from build123d import *

# Parameters (mm, degrees)
F0_W     = 43.18
F0_H     = 21.971
F0_W_2   = 40.64
F0_H_2   = 19.431
F1_DEPTH = 16.1544
F0_W_3   = 37.592
F0_H_3   = 16.383
F2_DEPTH = 1.27
F3_R     = 1.27
F4_R     = 1.27
F5_R     = 1.785938
F6_DEPTH = 7.62
F7_R     = 1.785938
F8_DEPTH = 7.62


with BuildPart() as f1:
    # F0 (on Front) → F1 (new body)
    with BuildSketch(Plane.XZ):
        Rectangle(F0_W, F0_H)
        Rectangle(F0_W_2, F0_H_2, mode=Mode.SUBTRACT)
    extrude(amount=F1_DEPTH)

    # F0 (on Front) → F2 (join)
    with BuildSketch(Plane.XZ):
        Rectangle(F0_W_2, F0_H_2)
        Rectangle(F0_W_3, F0_H_3, mode=Mode.SUBTRACT)
    extrude(amount=F2_DEPTH)

    # F3
    f3_edges = [f1.edges().sort_by_distance(p)[0] for p in [
        (-21.59, -8.0772, 10.9855),
        (-21.59, -8.0772, -10.9855),
        (21.59, -8.0772, -10.9855),
        (21.59, -8.0772, 10.9855),
    ]]
    fillet(f3_edges, radius=F3_R)

    # F4
    f4_edges = [f1.edges().sort_by_distance(p)[0] for p in [
        (0, 0, -10.9855),
    ]]
    fillet(f4_edges, radius=F4_R)

    # F5 (on face) → F6 (cut)
    with BuildSketch(Plane.YZ.offset(21.59)):
        with Locations((-8.7122, 0)):
            Circle(F5_R)
    extrude(amount=-F6_DEPTH, mode=Mode.SUBTRACT)

    # F7 (on face) → F8 (cut)
    with BuildSketch(Plane(origin=(-21.59, 0, 0), x_dir=(0, -1, 0), z_dir=(-1, 0, 0))):
        with Locations((8.7122, 0)):
            Circle(F7_R)
    extrude(amount=-F8_DEPTH, mode=Mode.SUBTRACT)


solid = f1.part
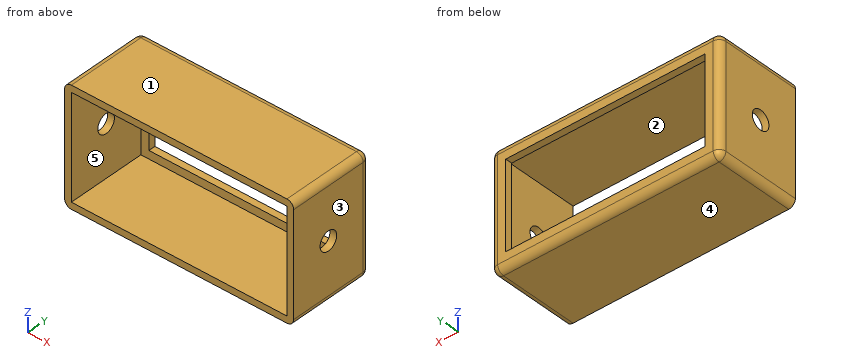
Work out the finished part from the listing and answer in its coordinate system (mm). Face numbers are marked on the shaded views. A direction names the side the tool comes from. Round coordinates to 2 decimals unless told otherwise and drop trailing zeros. Write each loop counter-clockwise with the first axis right and the second up, starting at its lowest first coordinate (ties: lowest second). Pieces come first, ordered by that corner, then holes. Notation, with made-up numbers: (53.25, 59.5) - (102.25, 59.5) arc R23 cw to (102.25, 95.5) - close; hole circle Ø4 at (-13, 55). An arc over 180 degrees is marked (long way). Answer in a Markdown table with one row per item. Add a question column.
1. For the marked faces 1 and 2, determine the directions among +Z, -Z, +X, -X, +Y, -Y from which every point of the face is accessible in a straight line to the end or side of a thin tool.
2. Find the intervals of material crossed by line 1 along Z through (x, y) = (-2, -15); line 2 along X through (y, z) = (-14.5, 2); line 3 along Z through (x, y) = (-14, -0.25), in increasing order. Write a range as from..to.
3. A cutting plane is placed at B-B, the plane z = 0. Determine the outline of the cut face in (x, y).
4. A cutting plane is placed at C-C, the plane x = -10. Determine the outline of the cut face in (y, z), and give its area (3 significant figures).
5. The mould has two halves that part along X. Classify the marked faces 3, 4 and 5: +X half, -X half, draft (parallel to the pull), parting line (faces both ways), or undercut.
6. Given pin 1 (5 mm diameter, centred on x = -4, z = 4.5, fed in from +Y), flat-ended and moving along its own axis, determine where the tip first touches the part or whether it passes through.
7. A cutting plane is placed at A-A, the plane y = -3. Determine the outline of the cut face in (x, z), and give its area (3 significant figures).
8. A cutting plane is placed at D-D, the plane y = -9. Determine the outline of the cut face in (x, z).
Worked out:
| question | item | result |
|---|---|---|
| 1 | face 1 | +Z, +X, -X, +Y, -Y |
| 1 | face 2 | -Y |
| 2 | line 1 | -10.99..-9.72, 9.72..10.99 |
| 2 | line 2 | -21.59..-20.32, 20.32..21.59 |
| 2 | line 3 | -10.47..-8.19, 8.19..10.47 |
| 3 | outline | (-21.59, -16.15) - (-20.32, -16.15) - (-20.32, -10.5) - (-21.59, -10.5) - close; (-21.59, -6.93) - (-20.32, -6.93) - (-20.32, -1.27) - (-18.8, -1.27) - (-18.8, 0) - (-20.32, 0) arc R1.27 ccw to (-21.59, -1.27) - close; (18.8, -1.27) - (20.32, -1.27) - (20.32, -6.93) - (21.59, -6.93) - (21.59, -1.27) arc R1.27 ccw to (20.32, 0) - (18.8, 0) - close; (20.32, -16.15) - (21.59, -16.15) - (21.59, -10.5) - (20.32, -10.5) - close |
| 4 | outline | (-16.15, -10.99) - (-1.27, -10.99) arc R1.27 ccw to (0, -9.72) - (0, -8.19) - (-1.27, -8.19) - (-1.27, -9.72) - (-16.15, -9.72) - close; (-16.15, 9.72) - (-1.27, 9.72) - (-1.27, 8.19) - (0, 8.19) - (0, 9.72) arc R1.27 ccw to (-1.27, 10.99) - (-16.15, 10.99) - close |
| 4 | area | 44.2 mm^2 |
| 5 | face 3 | +X half |
| 5 | face 4 | draft |
| 5 | face 5 | undercut |
| 6 | pin 1 | through |
| 7 | outline | (-21.59, -9.72) arc R1.27 ccw to (-20.32, -10.99) - (20.32, -10.99) arc R1.27 ccw to (21.59, -9.72) - (21.59, 9.72) arc R1.27 ccw to (20.32, 10.99) - (-20.32, 10.99) arc R1.27 ccw to (-21.59, 9.72) - close; hole (-20.32, -9.72) - (20.32, -9.72) - (20.32, 9.72) - (-20.32, 9.72) - close |
| 7 | area | 158 mm^2 |
| 8 | outline | (-21.59, -9.72) arc R1.27 ccw to (-20.32, -10.99) - (20.32, -10.99) arc R1.27 ccw to (21.59, -9.72) - (21.59, -1.76) - (20.32, -1.76) - (20.32, -9.72) - (-20.32, -9.72) - (-20.32, -1.76) - (-21.59, -1.76) - close; (-21.59, 1.76) - (-20.32, 1.76) - (-20.32, 9.72) - (20.32, 9.72) - (20.32, 1.76) - (21.59, 1.76) - (21.59, 9.72) arc R1.27 ccw to (20.32, 10.99) - (-20.32, 10.99) arc R1.27 ccw to (-21.59, 9.72) - close |
